Design review of the part shown in the three views and the two pictorial views. Dimensions are in mm from the part's minimum x, y and z. A direction names the side the tool comes from. Coordinates: 2 decimals unless noted, no trailing zeros. Order: outer loops, then holes, each group sorted by start corner. A loop starts at its lowest first (then second) coordinate and runs counter-clockwise, first axis right, second up. Notation, with made-up numbers: (84.5, -39.75) -> (100.5, -39.75) arc R28 cw to (100.5, -15.75) -> close; hole circle Ø7 at (63.5, 88.5). An arc over 180 degrees is marked (long way). Answer as a JSON object with one key per item and string values. Group by question number.
1) Wall thickness on L1, parallel to X at y = 3.5, z = 11; L2, parallel to Z at x = 36.5, y = 35.5; L3, parallel to Z at x = 39, y = 22: over which ranges is each line inside the solid? List them lowest first.
2) For pin 1 (4 mm diameter, centred on x = 57, z = 12, fed in from +Y); pin 2 (12 mm diameter, centred on x = 48, y = 24, fed in from -Z), all flat-tipped, find the tip position at first contact; note any pin that passes through.
3) Add section C-C, the plane x = 74. Write out the cut boundary in (y, z).
4) Add section D-D, the plane z = 10. Write out the cut boundary in (x, y).
5) Machinability: for the marked faces 4 and 5, which of the approach directions +Z, -Z, +X, -X, +Y, -Y give a long, thin tool a straight path to every point of the face, cutting with its end or side? Answer none if there is none.
6) Add section B-B, the plane y = 20. Write out the cut boundary in (x, z).
7) Add section A-A, the plane z = 18. Write out the cut boundary in (x, y).
8) Draft analysis for pull direction X (two halves, no side actions). For the marked faces 1, 2 and 3, state which applies: +X half, -X half, draft (parallel to the pull), parting line (faces both ways), or undercut.
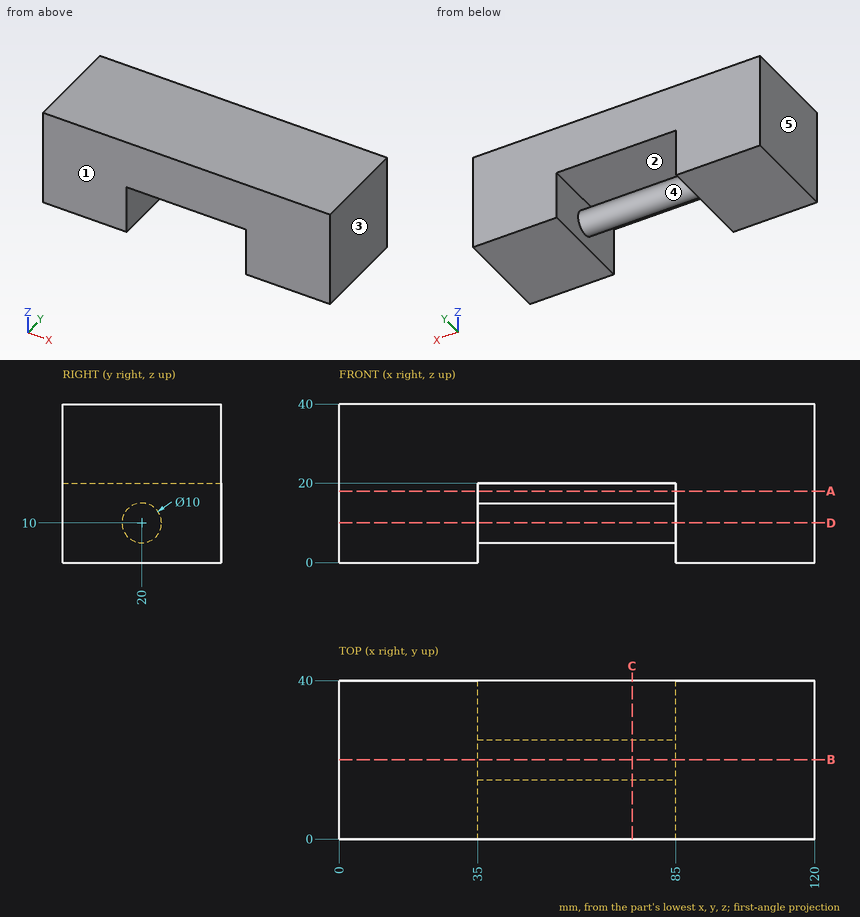
Output values:
{
 "1": {"L1": "x = 0 to 35, 85 to 120", "L2": "z = 20 to 40", "L3": "z = 5.42 to 14.58, 20 to 40"},
 "2": {"pin 1": "stops at y = 25", "pin 2": "stops at z = 5"},
 "3": {"outline": "(0, 20) -> (40, 20) -> (40, 40) -> (0, 40) -> close; circle Ø10 at (20, 10)"},
 "4": {"outline": "(0, 0) -> (35, 0) -> (35, 15) -> (85, 15) -> (85, 0) -> (120, 0) -> (120, 40) -> (85, 40) -> (85, 25) -> (35, 25) -> (35, 40) -> (0, 40) -> close"},
 "5": {"face 4": "none", "face 5": "+Z, -Z, -X, +Y, -Y"},
 "6": {"outline": "(0, 0) -> (35, 0) -> (35, 5) -> (85, 5) -> (85, 0) -> (120, 0) -> (120, 40) -> (0, 40) -> close; hole (35, 15) -> (85, 15) -> (85, 20) -> (35, 20) -> close"},
 "7": {"outline": "(0, 0) -> (35, 0) -> (35, 40) -> (0, 40) -> close; (85, 0) -> (120, 0) -> (120, 40) -> (85, 40) -> close"},
 "8": {"face 1": "draft", "face 2": "undercut", "face 3": "+X half"}
}
